The listing builds one solid part. Answer for the finished solid, in the listing's coordinates (mm). A direction names the side the tool comes from. Give positions to 0.01 mm unless a question says otherwise; leave off trailing zeros. Write each loop counter-clockwise with the first axis right and the second up, starting at its lowest first coordinate (ties: lowest second). Pieces come first, ordered by that corner, then holes. Notation, with made-up numbers: (58, -11) -> (85, -11) arc R33 cw to (85, 17) -> close; hole circle Ø6 at (28.25, 35). An arc over 180 degrees is marked (long way). Put each result on its own line as item: value. Start each with the question number.
1) A cutting plane is placed at D-D (z = 0.75). Write down the section's boundary in (x, y).
2) A cutting plane is placed at A-A (z = 4). Write down the section's boundary in (x, y).
3) For faces 1 (the cylindrical face through (6.335, 0.022, 2.799)), 2 (the flat face through (0.478, 0, -4)), determine the directions among +Z, -Z, +X, -X, +Y, -Y from which every point of the face is accessible in a straight line to the end or side of a thin tool.
4) For a pull along Z with two mould halves and no side action, classify faces 3 (the cylindrical face through (-2.127, -0.022, -4.076)), 4 (the cylindrical face through (0.27, 0.02, 6.66)), 5 (the flat face through (2.5, 1.588, 5.2)) as released by +Z, released by -Z, zero draft, split by the parting line, or undercut.
5) Flat-ended cylindrical pins translate along their axes: pin 1 Ø1.5 at (x, y) = (7.5, 0) entering from +Z; pin 2 Ø1.6 at (x, z) = (7.09, 2.11) entering from +Y. Find the tip coordinate at first contact, or state that the pin passes through.
6) A cutting plane is placed at B-B (y = -1.3). Give the number of separate pieces and of enclosed holes in the cut face, then the cut area to 3 significant figures.
7) Find the intervals of material crossed by line 1 along Z through (x, y) = (7, -0.7); line 2 along X through (y, z) = (-0.9, 4.25); line 3 along Z through (x, y) = (0.25, 0.95), in increasing order. Write a range as from..to.
8) A cutting plane is placed at C-C (x = -5.75). Write down the section's boundary in (y, z).
from build123d import *

# Parameters (mm, degrees)
F0_R     = 1.02362
F0_R_2   = 1.5875
F1_DEPTH = 1.5875


with BuildPart() as f1:
    # F0 (on Front) → F1 (new body, symmetric)
    with BuildSketch(Plane.XZ):
        with BuildLine():
            Line((-4.501804, -1.775407), (-4.471419, -3.052185))
            ThreePointArc((-4.471419, -3.052185), (-2.092182, -4.085642), (0.47765, -4.438859))
            Line((0.47765, -4.438859), (0.47765, -2.851359))
            Line((0.47765, -2.851359), (5.742792, -2.851359))
            ThreePointArc((5.742792, -2.851359), (1.310194, 14.574686), (-6.089304, -1.813188))
            Line((-6.089304, -1.813188), (-4.501804, -1.775407))
        make_face()
        with Locations((7.089037, 2.107543)):
            Circle(F0_R, mode=Mode.SUBTRACT)
        with Locations((0.47765, 5.086141)):
            Circle(F0_R_2, mode=Mode.SUBTRACT)
    extrude(amount=F1_DEPTH, both=True)


solid = f1.part
Reply:
1. outline: (-8, -1.59) -> (8.96, -1.59) -> (8.96, 1.59) -> (-8, 1.59) -> close
2. outline: (-8.99, -1.59) -> (-0.68, -1.59) -> (-0.68, 1.59) -> (-8.99, 1.59) -> close; (1.64, -1.59) -> (9.94, -1.59) -> (9.94, 1.59) -> (1.64, 1.59) -> close
3. face 1: +Y, -Y
3. face 2: -Z, +X, +Y, -Y
4. face 3: released by -Z
4. face 4: undercut
4. face 5: zero draft
5. pin 1: stops at z = 12.25
5. pin 2: passes through
6. separate pieces: 1
6. enclosed holes: 2
6. area: 267 mm2
7. line 1: z = -1.86..1.09, 3.13..12.03
7. line 2: x = -9.01..-0.87, 1.83..9.97
7. line 3: z = -4.44..3.52, 6.66..14.61
8. outline: (-1.59, -1.81) -> (1.59, -1.81) -> (1.59, 12.29) -> (-1.59, 12.29) -> close
